```python
from build123d import *

# Parameters (mm, degrees)
SKETCH_1_W          = 104.4
SKETCH_1_H          = 106.6
EXTRUDE_1_DEPTH     = 1
SKETCH_2_W          = 101.7
SKETCH_2_H          = 103.9
SKETCH_2_W_2        = 100.1
SKETCH_2_H_2        = 102.3
EXTRUDE_2_DEPTH     = 2.5
SKETCH_4_R          = 2.7
CUT_EXTRUDE_1_DEPTH = 75.685875505
EXTRUDE_3_DEPTH     = 2.5
FILLET_1_R          = 1
FILLET_2_R          = 0.5
CHAMFER_1_SIZE      = 1
SKETCH_6_R          = 2
SKETCH_6_R_2        = 0.95
EXTRUDE_4_DEPTH     = 0.8
EXTRUDE_START       = -0.8
SKETCH_7_R          = 2
SKETCH_7_R_2        = 0.95
EXTRUDE_5_DEPTH     = 0.8
SKETCH_8_R          = 0.95
CUT_EXTRUDE_2_DEPTH = 0.8
CUT_EXTRUDE_START   = -0.8
SKETCH_9_R          = 0.95
CUT_EXTRUDE_3_DEPTH = 0.8
FILLET_3_R          = 1
EXTRUDE_START_2     = -3
SKETCH_10_R         = 0.95
EXTRUDE_6_DEPTH     = 3
SKETCH_11_R         = 0.95
EXTRUDE_7_DEPTH     = 3


with BuildPart() as part:
    # 草图1 → 凸台-拉伸1 (new body)
    with BuildSketch(Plane(origin=(0, 0, 0), x_dir=(1, 0, 0), z_dir=(0, 1, 0))):
        Rectangle(SKETCH_1_W, SKETCH_1_H)
    extrude(amount=EXTRUDE_1_DEPTH)

    # 草图2 → 凸台-拉伸2 (add)
    with BuildSketch(Plane.XZ):
        Rectangle(SKETCH_2_W, SKETCH_2_H)
        Rectangle(SKETCH_2_W_2, SKETCH_2_H_2, mode=Mode.SUBTRACT)
    extrude(amount=EXTRUDE_2_DEPTH)

    # 草图4 → 切除-拉伸1 (cut, through all)
    with BuildSketch(Plane(origin=(0, 1, 0), x_dir=(1, 0, 0), z_dir=(0, 1, 0))):
        with Locations(Location((47.5, 45.95, 0), (0, 0, 270))):
            Circle(SKETCH_4_R)
        with Locations(Location((-47.5, 45.95, 0), (0, 0, 270))):
            Circle(SKETCH_4_R)
        with Locations(Location((-47.5, -45.925, 0), (0, 0, 270))):
            Circle(SKETCH_4_R)
        with Locations(Location((47.5, -45.925, 0), (0, 0, 270))):
            Circle(SKETCH_4_R)
    extrude(amount=-CUT_EXTRUDE_1_DEPTH, mode=Mode.SUBTRACT)

    # 草图5 → 凸台-拉伸3 (add)
    with BuildSketch(Plane.XZ):
        Polygon((0.4, 51.15), (-0.4, 51.15), (-0.4, 0.4), (-50.05, 0.4), (-50.05, -0.4), (-0.4, -0.4), (-0.4, -51.15), (0.4, -51.15), (0.4, -0.4), (50.05, -0.4), (50.05, 0.4), (0.4, 0.4), align=None)
    extrude(amount=EXTRUDE_3_DEPTH)

    # 圆角1
    fillet_1_edges = [part.edges().sort_by_distance(p)[0] for p in [
        (-0.4, -1.25, 0.4),
        (-50.05, -1.25, 0.4),
        (-50.05, -1.25, -0.4),
        (50.05, -1.25, -0.4),
        (0.4, -1.25, 0.4),
        (50.05, -1.25, 0.4),
        (0.4, -1.25, -0.4),
        (0.4, -1.25, -51.15),
        (-0.4, -1.25, -51.15),
        (-0.4, -1.25, -0.4),
        (0.4, -1.25, 51.15),
        (-0.4, -1.25, 51.15),
        (50.05, -1.25, -51.15),
        (50.05, -1.25, 51.15),
        (-50.05, -1.25, 51.15),
        (-50.05, -1.25, -51.15),
        (50.05, -1.25, 46.812411967),
        (50.05, -1.25, 45.037588033),
        (-50.05, -1.25, 45.037588033),
        (-50.05, -1.25, 46.812411967),
        (-50.05, -1.25, -46.837411967),
        (-50.05, -1.25, -45.062588033),
        (50.05, -1.25, -45.062588033),
        (50.05, -1.25, -46.837411967),
    ]]
    fillet(fillet_1_edges, radius=FILLET_1_R)

    # 圆角2
    fillet_2_edges = [part.edges().sort_by_distance(p)[0] for p in [
        (-50.85, -1.25, -51.95),
        (50.85, -1.25, -51.95),
        (50.85, -1.25, 51.95),
        (-50.85, -1.25, 51.95),
    ]]
    fillet(fillet_2_edges, radius=FILLET_2_R)

    # 倒角1
    chamfer_1_edges = [part.edges().sort_by_distance(p)[0] for p in [
        (52.2, 0.5, 53.3),
        (-52.2, 0.5, 53.3),
        (-52.2, 0.5, -53.3),
        (52.2, 0.5, -53.3),
    ]]
    chamfer(chamfer_1_edges, length=CHAMFER_1_SIZE)

    # 草图6 → 凸台-拉伸4 (add)
    # profile 1 of 2: a face of its own
    with BuildSketch(Plane(origin=(50.85, 0, 0), x_dir=(0, 0, -1), z_dir=(1, 0, 0))):
        with Locations((-40.3, -2)):
            Circle(SKETCH_6_R)
        with Locations((-40.3, -2)):
            Circle(SKETCH_6_R_2, mode=Mode.SUBTRACT)
    # profile 2 of 2: a face of its own
    with BuildSketch(Plane(origin=(50.85, 0, 0), x_dir=(0, 0, -1), z_dir=(1, 0, 0))):
        with Locations((40.3, -2)):
            Circle(SKETCH_6_R)
        with Locations((40.3, -2)):
            Circle(SKETCH_6_R_2, mode=Mode.SUBTRACT)
    extrude(amount=-EXTRUDE_4_DEPTH)

    # 草图7 → 凸台-拉伸5 (add)
    # profile 1 of 2: a face of its own
    with BuildSketch(Plane.ZY.offset(50.85).offset(EXTRUDE_START)):
        with Locations((-40.3, -2)):
            Circle(SKETCH_7_R)
        with Locations((-40.3, -2)):
            Circle(SKETCH_7_R_2, mode=Mode.SUBTRACT)
    # profile 2 of 2: a face of its own
    with BuildSketch(Plane.ZY.offset(50.85).offset(EXTRUDE_START)):
        with Locations((40.3, -2)):
            Circle(SKETCH_7_R)
        with Locations((40.3, -2)):
            Circle(SKETCH_7_R_2, mode=Mode.SUBTRACT)
    extrude(amount=EXTRUDE_5_DEPTH)

    # 草图8 → 切除-拉伸2 (cut)
    with BuildSketch(Plane(origin=(50.85, 0, 0), x_dir=(0, 0, -1), z_dir=(1, 0, 0))):
        with Locations(Location((40.3, -2, 0), (0, 0, 180))):
            Circle(SKETCH_8_R)
        with Locations((-40.3, -2)):
            Circle(SKETCH_8_R)
    extrude(amount=-CUT_EXTRUDE_2_DEPTH, mode=Mode.SUBTRACT)

    # 草图9 → 切除-拉伸3 (cut)
    with BuildSketch(Plane.ZY.offset(50.85).offset(CUT_EXTRUDE_START)):
        with Locations(Location((40.3, -2, 0), (0, 0, 180))):
            Circle(SKETCH_9_R)
        with Locations((-40.3, -2)):
            Circle(SKETCH_9_R)
    extrude(amount=CUT_EXTRUDE_3_DEPTH, mode=Mode.SUBTRACT)

    # 圆角3
    fillet_3_edges = [part.edges().sort_by_distance(p)[0] for p in [
        (50.45, -2.5, 38.363508327),
        (50.45, -2.5, 42.236491673),
        (50.45, -2.5, -42.236491673),
        (50.45, -2.5, -38.363508327),
        (-50.45, -2.5, -38.363508327),
        (-50.45, -2.5, -42.236491673),
        (-50.45, -2.5, 42.236491673),
        (-50.45, -2.5, 38.363508327),
    ]]
    fillet(fillet_3_edges, radius=FILLET_3_R)

    # 草图10 → 凸台-拉伸6 (add)
    # profile 1 of 2: a face of its own
    with BuildSketch(Plane.ZY.offset(50.85).offset(EXTRUDE_START_2)):
        with BuildLine():
            Line((-42.3, -2), (-42.3, 0))
            Line((-42.3, 0), (-38.3, 0))
            Line((-38.3, 0), (-38.3, -2))
            ThreePointArc((-38.3, -2), (-40.3, -4), (-42.3, -2))
        make_face()
        with Locations((-40.3, -2)):
            Circle(SKETCH_10_R, mode=Mode.SUBTRACT)
    # profile 2 of 2: a face of its own
    with BuildSketch(Plane.ZY.offset(50.85).offset(EXTRUDE_START_2)):
        with BuildLine():
            Line((38.3, -2), (38.3, 0))
            Line((38.3, 0), (42.3, 0))
            Line((42.3, 0), (42.3, -2))
            ThreePointArc((42.3, -2), (40.3, -4), (38.3, -2))
        make_face()
        with Locations(Location((40.3, -2, 0), (0, 0, 180))):
            Circle(SKETCH_10_R, mode=Mode.SUBTRACT)
    extrude(amount=EXTRUDE_6_DEPTH)

    # 草图11 → 凸台-拉伸7 (add)
    # profile 1 of 2: a face of its own
    with BuildSketch(Plane(origin=(50.85, 0, 0), x_dir=(0, 0, -1), z_dir=(1, 0, 0))):
        with BuildLine():
            Line((-38.3, -2), (-38.3, 0))
            Line((-38.3, 0), (-42.3, 0))
            Line((-42.3, 0), (-42.3, -2))
            ThreePointArc((-42.3, -2), (-40.3, -4), (-38.3, -2))
        make_face()
        with Locations((-40.3, -2)):
            Circle(SKETCH_11_R, mode=Mode.SUBTRACT)
    # profile 2 of 2: a face of its own
    with BuildSketch(Plane(origin=(50.85, 0, 0), x_dir=(0, 0, -1), z_dir=(1, 0, 0))):
        with BuildLine():
            Line((42.3, -2), (42.3, 0))
            Line((42.3, 0), (38.3, 0))
            Line((38.3, 0), (38.3, -2))
            ThreePointArc((38.3, -2), (40.3, -4), (42.3, -2))
        make_face()
        with Locations((40.3, -2)):
            Circle(SKETCH_11_R, mode=Mode.SUBTRACT)
    extrude(amount=-EXTRUDE_7_DEPTH)


solid = part.part
```
CAD build for the part. Positions are in the model's coordinates, mm. A direction names the side the tool comes from. Coordinates: 2 decimals unless noted, no trailing zeros. Loops run counter-clockwise (first coordinate to the right, second up) from the corner with the lowest first, then second, coordinate; pieces in that order, holes last. Notation, with made-up numbers: (24.5, 10) - (42.5, 10) arc R32 cw to (42.5, 42) - close; hole circle Ø3 at (69, 78). An arc over 180 degrees is marked (long way). Return JSON: item names as keys, results as strings.
1. Probe L1, parallel to X at y = -1.5, z = -45.95; L2, parallel to X at y = -0.55, z = 5; L3, parallel to Z at x = -47.5, y = -1.35. List the from-to ranges inside material, lowest first. Write a range as from..to.
Result:
{"L1": "x = -50.85..-50.2, -0.4..0.4, 50.2..50.85", "L2": "x = -50.85..-50.05, -0.4..0.4, 50.05..50.85", "L3": "z = -51.95..-51.15, -0.4..0.4, 51.15..51.95"}
2. 3-axis set-ups, long thin cutter, end or side, ignore diameter. For faces 1 (the cylindrical face through (50.177, 0.052, -46.301)), 2 (the flat face through (25, -1, 51.15)): which of +Z, -Z, +X, -X, +Y, -Y reach the whole face in a straight line?
Result:
{"face 1": "+Y, -Y", "face 2": "-Y"}
3. Band-saw the part on B-B (z = -9). Give the cut face in (x, y), and give its area (3 significant figures).
Result:
{"outline": "(-52.2, 0) - (-50.85, 0) - (-50.85, -2.5) - (-50.05, -2.5) - (-50.05, 0) - (-0.4, 0) - (-0.4, -2.5) - (0.4, -2.5) - (0.4, 0) - (50.05, 0) - (50.05, -2.5) - (50.85, -2.5) - (50.85, 0) - (52.2, 0) - (52.2, 1) - (-52.2, 1) - close", "area": "110 mm2"}
4. Band-saw the part on A-A (x = 12). Give the cut face in (y, z).
Result:
{"outline": "(-2.5, -51.95) - (0, -51.95) - (0, -53.3) - (1, -53.3) - (1, 53.3) - (0, 53.3) - (0, 51.95) - (-2.5, 51.95) - (-2.5, 51.15) - (0, 51.15) - (0, 0.4) - (-2.5, 0.4) - (-2.5, -0.4) - (0, -0.4) - (0, -51.15) - (-2.5, -51.15) - close"}
5. Drop flat-ended pins along their axis: pin 1 (6 mm diameter, centred on x = -11.5, z = -2, fed in from -Y); pin 2 (1.5 mm diameter, centred on x = -1, y = -1.5, fed in from -Z); pin 3 (1 mm diameter, centred on y = -1, z = 1.5, fed in from +X). Give the stop position or say it passes through.
Result:
{"pin 1": "stops at y = -2.5", "pin 2": "stops at z = -51.95", "pin 3": "stops at x = 50.85"}
6. Mould opens along Z. For faces 3 (the flat face through (-1, -1, -51.95)), 4 (the cylindrical face through (-50.136, 0.052, 45.34)), 5 (the flat face through (-47.85, -1, 41)) say: released by +Z, released by -Z, zero draft, split by the parting line, or undercut.
Result:
{"face 3": "released by -Z", "face 4": "undercut", "face 5": "undercut"}
